Read the model definition and answer for the solid it produces. Units are mm, in the model's axes. A direction names the side the tool comes from. Coordinates: 2 decimals unless noted, no trailing zeros. Loops run counter-clockwise (first coordinate to the right, second up) from the corner with the lowest first, then second, coordinate; pieces in that order, holes last. Notation, with made-up numbers: (38.25, -15.5) - (44.25, -15.5) arc R23 ccw to (44.25, 3.5) - close; hole circle Ø4 at (-39.5, -31.5). An arc over 180 degrees is marked (long way). Use one line per item in the form item = value. Start each with the question number.
1) A cutting plane is placed at A-A (y = 5). Give the vertices of the cut face in (x, z).
2) A cutting plane is placed at B-B (x = 10). Give the vertices of the cut face in (y, z), and give its area (3 significant figures).
3) Which of the six approach directions +Z, -Z, +X, -X, +Y, -Y give full straight-line access (tool end or side, diameter ignored) to faces 4 (the face through (13, 10, 0)), 5 (the face through (84.75, 10, -160))?
4) Consider line 1 (Y direction, x = 10, z = -1.6); line 2 (Z direction, x = 13, y = 9); line 3 (Z direction, x = 39.5, y = 17.5). Determine where each line is inside the solid, lowest interval first.
5) The mould has two halves that part along Y. Classify faces 1 (the face through (69, 20, -97)), 2 (the face through (9.46, 7.56, -0.99)), 3 (the face through (86.75, 10, -160)): released by +Y, released by -Y, zero draft, split by the parting line, or undercut.
6) Each of these flat-tipped pins is pushed along its axis until it touches: P1, Ø10, axis at x = 14.5, y = 13.5, coming from the -Z side; P2, Ø8, axis at x = 75, y = 5.5, coming from the -Z side; P3, Ø12, axis at x = 21.5, y = 14.5, coming from the -Z side. Where does it stop, or does it pass through?
7) A cutting plane is placed at C-C (y = 16.25). Give the vertices of the cut face in (x, z).
8) A cutting plane is placed at D-D (z = -110). Give the vertices of the cut face in (x, y).
from build123d import *

# Parameters (mm, degrees)
BOSS_EXTRUDE1_DEPTH  = 20
CONVERT_SOLID2_DEPTH = 20
SKETCH8_R            = 2.5
CUT_EXTRUDE1_DEPTH   = 20
CUT_EXTRUDE2_DEPTH   = 10


# Read off the part's stored shape, not the designer's step: Convert-Solid2
with BuildPart() as part:
    # Sketch1 → Boss-Extrude1 (new body)
    with BuildSketch(Plane(origin=(0, 0, 0), x_dir=(1, 0, 0), z_dir=(0, 1, 0))):
        Polygon((0, 0), (30, 0), (86.75, 140), (86.75, 180), (81.75, 180), (81.75, 140.974868952), (26.631615621, 5), (0, 5), align=None)
    extrude(amount=BOSS_EXTRUDE1_DEPTH)

    # Convert-Solid2 outline → Convert-Solid2 (cut)
    with BuildSketch(Plane(origin=(0, 0, 0), x_dir=(1, 0, 0), z_dir=(0, 1, 0))):
        with BuildLine():
            Line((30, 0), (31.51846779, 3.745999834))
            ThreePointArc((31.51846779, 3.745999834), (29.310251306, 1.023856865), (25.957938746, 0))
            Line((25.957938746, 0), (30, 0))
        make_face()
        with BuildLine():
            ThreePointArc((86.75, 141.169842742), (86.639107499, 140.021621131), (86.310529044, 138.915842576))
            Line((86.310529044, 138.915842576), (86.75, 140))
            Line((86.75, 140), (86.75, 141.169842742))
        make_face()
        with BuildLine():
            Line((0, 5), (0, 2))
            Line((0, 2), (25.957938746, 2))
            ThreePointArc((25.957938746, 2), (28.192813786, 2.682571243), (29.664958108, 4.497333223))
            Line((29.664958108, 4.497333223), (84.457019363, 139.667175965))
            ThreePointArc((84.457019363, 139.667175965), (84.676071666, 140.404361668), (84.75, 141.169842742))
            Line((84.75, 141.169842742), (84.75, 180))
            Line((84.75, 180), (81.75, 180))
            Line((81.75, 180), (81.75, 140.974868952))
            Line((81.75, 140.974868952), (26.631615621, 5))
            Line((26.631615621, 5), (0, 5))
        make_face()
    extrude(amount=CONVERT_SOLID2_DEPTH, mode=Mode.SUBTRACT)

    # Sketch8 → Cut-Extrude1 (cut)
    with BuildSketch(Plane.XY):
        with Locations((10, 10)):
            Circle(SKETCH8_R)
    extrude(amount=-CUT_EXTRUDE1_DEPTH, mode=Mode.SUBTRACT)

    # Sketch9 → Cut-Extrude2 (cut)
    with BuildSketch(Plane(origin=(86.75, 0, -320.372504423), x_dir=(0, 0, 1), z_dir=(-1, 0, 0))):
        with BuildLine():
            Line((145.372504423, 7.5), (165.372504423, 7.5))
            ThreePointArc((165.372504423, 7.5), (167.872504423, 5), (165.372504423, 2.5))
            Line((165.372504423, 2.5), (145.372504423, 2.5))
            ThreePointArc((145.372504423, 2.5), (142.872504423, 5), (145.372504423, 7.5))
        make_face()
    extrude(amount=CUT_EXTRUDE2_DEPTH, mode=Mode.SUBTRACT)


solid = part.part
Found:
q1.outline = (0, -2) - (25.96, -2) arc R4 cw to (29.66, -4.5) - (84.46, -139.67) arc R4 cw to (84.75, -141.17) - (84.75, -152.5) - (86.75, -152.5) - (86.75, -141.17) arc R6 ccw to (86.31, -138.92) - (31.52, -3.75) arc R6 ccw to (25.96, 0) - (0, 0) - close; (84.75, -180) - (86.75, -180) - (86.75, -177.5) - (84.75, -177.5) - close
q2.outline = (0, -2) - (7.5, -2) - (7.5, 0) - (0, 0) - close; (12.5, -2) - (20, -2) - (20, 0) - (12.5, 0) - close
q2.area = 30.0 mm^2
q3.face_4 = +Z, +X, -X, +Y, -Y
q3.face_5 = -Z, -X, +Y, -Y
q4.line_1 = 0 to 7.5, 12.5 to 20
q4.line_2 = -2 to 0
q4.line_3 = -28.76 to -23.44
q5.face_1 = released by +Y
q5.face_2 = undercut
q5.face_3 = zero draft
q6.P1 = -2
q6.P2 = -126.2
q6.P3 = -2.31
q7.outline = (0, -2) - (25.96, -2) arc R4 cw to (29.66, -4.5) - (84.46, -139.67) arc R4 cw to (84.75, -141.17) - (84.75, -180) - (86.75, -180) - (86.75, -141.17) arc R6 ccw to (86.31, -138.92) - (31.52, -3.75) arc R6 ccw to (25.96, 0) - (0, 0) - close
q8.outline = (72.43, 0) - (74.59, 0) - (74.59, 20) - (72.43, 20) - close
